Check sheet for the modelled part. Datum: model origin and axes. Units: mm. A direction names the side the tool comes from. Coordinates: 2 decimals unless noted, no trailing zeros. Loops run counter-clockwise (first coordinate to the right, second up) from the corner with the lowest first, then second, coordinate; pieces in that order, holes last. Notation, with made-up numbers: M -11.5,49.25 L 18.5,49.25 A24 ccw 18.5,66.25 Z; hole C 67.25,21 d10. An arc over 180 degrees is marked long. Answer in a Markdown table with one row per item. Add a question column.
```python
from build123d import *

# Parameters (mm, degrees)
F0_R     = 0.84
F1_DEPTH = 29.6
F2_W     = 0.9
F2_H     = 0.6
F4_R     = 0.455
F5_DEPTH = 8.38
F6_R     = 0.45


with BuildPart() as f1:
    # F0 (on Top) → F1 (new body)
    with BuildSketch(Plane.XY):
        Circle(F0_R)
    extrude(amount=F1_DEPTH)

    # F2 (on Right) → F3 (revolve)
    with BuildSketch(Plane.YZ):
        with Locations((0.45, 7.32)):
            Rectangle(F2_W, F2_H)
    revolve(axis=Axis((0, 0, 7.32), (0, 0, 1)))

    # F4 (on Top) → F5 (join)
    with BuildSketch(Plane.XY):
        Circle(F4_R)
    extrude(amount=-F5_DEPTH)

    # F6
    f6_edges = [f1.edges().sort_by_distance(p)[0] for p in [
        (-0.455, 0, -8.38),
    ]]
    fillet(f6_edges, radius=F6_R)


solid = f1.part
```
Q1. Thickness scan on L1, parallel to Z at x = 0.5, y = -0.1; L2, parallel to Y at x = -0.05, z = 2.5. Record the ranges inside material, lowest first.
Q2. Access from +Z, -Z, +X, -X, +Y, -Y to the whole of each face (thin tool, end or side, straight path). Record for faces 1 (the face through (-0.27, 0.86, 7.32)), 2 (the face through (0.388, -0.745, 18.456)), 3 (the face through (0.388, -0.745, 3.461)).
Q3. Cross-section at B-B (z = -3). Record the cut outline in (x, y) (3 decimals).
Q4. Cross-section at A-A (z = 4). Record the cut outline in (x, y).
Answer key:
| question | item | result |
|---|---|---|
| 1 | L1 | 0 to 29.6 |
| 1 | L2 | -0.84 to 0.84 |
| 2 | face 1 | +Z, -Z |
| 2 | face 2 | +Z |
| 2 | face 3 | -Z |
| 3 | outline | C 0,0 d0.91 |
| 4 | outline | C 0,0 d1.68 |
